from build123d import *

# Parameters (mm, degrees)
BOSS_EXTRUDE1_DEPTH = 5


with BuildPart() as part:
    # Sketch1 → Boss-Extrude1 (new body)
    with BuildSketch(Plane(origin=(0, 0, 0), x_dir=(1, 0, 0), z_dir=(0, 1, 0))):
        with BuildLine():
            Line((0, -9.994125046), (0, -14.994125046))
            Line((0, -14.994125046), (3.808365199, -9.240312874))
            Line((3.808365199, -9.240312874), (5.72178236, -13.859710537))
            Line((5.72178236, -13.859710537), (7.038364429, -7.086482971))
            Line((7.038364429, -7.086482971), (10.573898335, -10.622016877))
            Line((10.573898335, -10.622016877), (9.186628177, -3.803366209))
            Line((9.186628177, -3.803366209), (13.858414609, -5.73848351))
            Line((13.858414609, -5.73848351), (9.999983576, -0.018124259))
            ThreePointArc((9.999983576, -0.018124259), (9.999995894, -0.009062133), (10, 0))
            Line((10, 0), (15, 0))
            Line((15, 0), (9.246512341, 3.808150408))
            Line((9.246512341, 3.808150408), (13.865910003, 5.72156757))
            Line((13.865910003, 5.72156757), (7.106491915, 7.035465347))
            Line((7.106491915, 7.035465347), (10.642025821, 10.570999253))
            Line((10.642025821, 10.570999253), (3.914062891, 9.202179725))
            Line((3.914062891, 9.202179725), (5.827480053, 13.821577387))
            Line((5.827480053, 13.821577387), (0.160205895, 9.998952701))
            ThreePointArc((0.160205895, 9.998952701), (0.080105518, 9.999915207), (0, 10.000236049))
            Line((0, 10.000236049), (0, 15.000236049))
            Line((0, 15.000236049), (-3.808365199, 9.246423877))
            Line((-3.808365199, 9.246423877), (-5.72178236, 13.86582154))
            Line((-5.72178236, 13.86582154), (-7.03571003, 7.10624967))
            Line((-7.03571003, 7.10624967), (-10.571243936, 10.641783576))
            Line((-10.571243936, 10.641783576), (-9.202378572, 3.913595357))
            Line((-9.202378572, 3.913595357), (-13.821776235, 5.827012519))
            Line((-13.821776235, 5.827012519), (-9.963345201, 0.106653268))
            ThreePointArc((-9.963345201, 0.106653268), (-9.963773316, 0.053327398), (-9.963916023, 0))
            Line((-9.963916023, 0), (-14.963916023, 0))
            Line((-14.963916023, 0), (-9.21010385, -3.808365199))
            Line((-9.21010385, -3.808365199), (-13.829501513, -5.72178236))
            Line((-13.829501513, -5.72178236), (-7.056273947, -7.038364429))
            Line((-7.056273947, -7.038364429), (-10.591807853, -10.573898335))
            Line((-10.591807853, -10.573898335), (-3.830327391, -9.198259587))
            Line((-3.830327391, -9.198259587), (-5.743744553, -13.81765725))
            Line((-5.743744553, -13.81765725), (0, -9.994125046))
        make_face()
        with BuildLine():
            Line((-2, -4.8), (-2, -2.3))
            Line((-2, -2.3), (2, -2.3))
            Line((2, -2.3), (2, -4.8))
            ThreePointArc((2, -4.8), (0, 5.2), (-2, -4.8))
        make_face(mode=Mode.SUBTRACT)
    extrude(amount=BOSS_EXTRUDE1_DEPTH)


solid = part.part
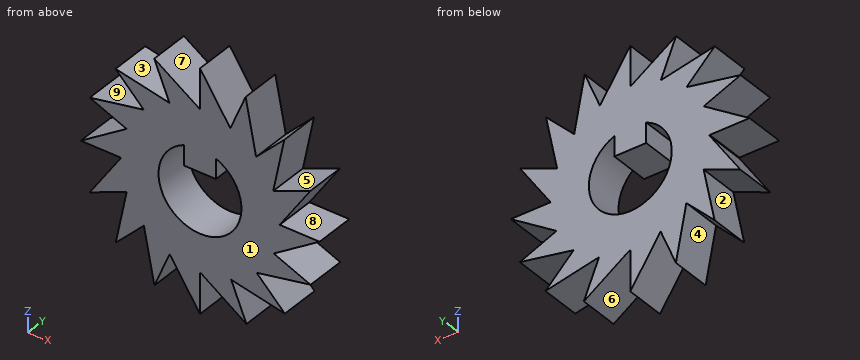
Verification items for the finished model (mm, model axes). Face numbers are marked on the shaded views. A direction names the side the tool comes from. Give positions to 0.01 mm unless a question says otherwise; leave off trailing zeros. Write each loop counter-clockwise with the first axis right and the second up, starting at its lowest first coordinate (ties: lowest second). Pieces come first, ordered by that corner, then holes. Notation, with made-up numbers: M 39.5,30.5 L 75.5,30.5 A23 ccw 75.5,45.5 Z; hole C -31,22 d9. An arc over 180 degrees is marked long. Put each result on its own line as item: value. Start each with the question number.
1. Section check B-B (x = 12.75). Record the cut outline in (y, z).
2. Section check C-C (z = -8.5). Record the cut outline in (x, y), and give its area (3 significant figures).
3. Set-up check for the marked faces 5, 6, 7, 8 and 9: record each of +Z, -Z, +X, -X, +Y, -Y from which the full face is reachable in a straight line by a thin tool's end or side.
4. Draft check along Z on the marked faces 1, 2, 3 and 4. Enter one of: +Z half, -Z half, draft (parallel to the pull), parting line (faces both ways), or undercut.
5. Section check A-A (z = -11.75). Record the cut outline in (x, y).
6. Scan lines: line 1 along X through (y, z) = (2.6, 4); line 2 along X through (y, z) = (4.15, 2.75); line 3 along Z through (x, y) = (-11.75, 1.1). Record each from-to range of solid material in increasing order. Write a range as [from, to].
7. Go/stop test with flat-tipped pins: pin 1 Ø1.5 at (x, y) = (-10, 1) entering from +Z; pin 2 Ø0.8 at (y, z) = (2.5, 3.5) entering from +X; pin 3 Ø4 at (x, z) = (4, 8.5) entering from -Y; pin 4 Ø1.3 at (y, z) = (2.5, 3.5) entering from -X. Record where each tip stops, or that it passes through.
Answer list:
1. outline: M 0,-5.94 L 5,-5.94 L 5,-5.26 L 0,-5.26 Z; M 0,-1.49 L 5,-1.49 L 5,0 L 0,0 Z; M 0,4.1 L 5,4.1 L 5,5.28 L 0,5.28 Z
2. outline: M -10.14,0 L -8.43,0 L -8.43,5 L -10.14,5 Z; M -6.76,0 L 8.57,0 L 8.57,5 L -6.76,5 Z
2. area: 85.2 mm2
3. face 5: +Y, -Y
3. face 6: -Z, +Y, -Y
3. face 7: +Z, +Y, -Y
3. face 8: +X, +Y, -Y
3. face 9: -X, +Y, -Y
4. face 1: draft
4. face 2: undercut
4. face 3: undercut
4. face 4: -Z half
5. outline: M -6.13,0 L -4.85,0 L -4.85,5 L -6.13,5 Z; M -2.15,0 L 0,0 L 0,5 L -2.15,5 Z; M 2.76,0 L 4.97,0 L 4.97,5 L 2.76,5 Z
6. line 1: [-9.67, -3.32], [-2, 2], [3.32, 9.23], [9.66, 12.69]
6. line 2: [-10.81, -4.41], [-2, 2], [4.41, 11.84]
6. line 3: [-4.97, -2.76], [0, 2.13], [4.86, 6.13]
7. pin 1: z = 10.57
7. pin 2: x = 12.62
7. pin 3: y = 0
7. pin 4: x = -10.66
